CAD build for the part. Positions are in the model's coordinates, mm. A direction names the side the tool comes from. Round coordinates to 2 decimals unless told otherwise and drop trailing zeros. Loops run counter-clockwise (first coordinate to the right, second up) from the corner with the lowest first, then second, coordinate; pieces in that order, holes last. Notation, with made-up numbers: M 16,-26 L 37,-26 A19 cw 37,-20 Z; hole C 45,54 d8. An arc over 180 degrees is marked long. Put each result on its own line as item: value. Start each with the question number.
from build123d import *

# Parameters (mm, degrees)
F0_W     = 59.6908442676
F0_H     = 73.2762925327
F0_W_2   = 45.3756786883
F1_DEPTH = 38.1
F3_DEPTH = 76.2
F4_W     = 20.4342082143
F4_H     = 8.8877151668
F5_DEPTH = 76.2
F6_W     = 27.9634296894
F6_H     = 14.7078186274
F7_DEPTH = 25.4
F8_R     = 4.8926994205
F8_R_2   = 4.9486448894
F8_R_3   = 4.9129402175
F8_R_4   = 5.3604581345
F9_DEPTH = 76.2


with BuildPart() as f1:
    # F0 (on Top) → F1 (new body)
    with BuildSketch(Plane.XY):
        with Locations((-29.8454221338, -36.6381462663)):
            Rectangle(F0_W, F0_H)
        with Locations((22.6878393441, -36.6381462663)):
            Rectangle(F0_W_2, F0_H)
    extrude(amount=F1_DEPTH)

    # F2 (on Front) → F3 (cut)
    with BuildSketch(Plane.XZ):
        Polygon((-9.0658813715, 42.4513481557), (46.1928248405, 0), (48.2074655592, 0), (48.2074655592, 42.4513481557), align=None)
    extrude(amount=F3_DEPTH, mode=Mode.SUBTRACT)

    # F4 (on face) → F5 (cut)
    with BuildSketch(Plane(origin=(-59.6908442676, 0, 0), x_dir=(0, -1, 0), z_dir=(-1, 0, 0))):
        with Locations((37.7025529742, 33.6561424166)):
            Rectangle(F4_W, F4_H)
    extrude(amount=-F5_DEPTH, mode=Mode.SUBTRACT)

    # F6 (on face) → F7 (cut)
    with BuildSketch(Plane(origin=(0, 0, 0), x_dir=(1, 0, 0), z_dir=(0, 0, -1))):
        with Locations((31.3939638436, 65.922383219)):
            Rectangle(F6_W, F6_H)
    extrude(amount=-F7_DEPTH, mode=Mode.SUBTRACT)

    # F8 (on face) → F9 (cut)
    with BuildSketch(Plane(origin=(0, 0, 0), x_dir=(1, 0, 0), z_dir=(0, 0, -1))):
        with Locations((12.5195495784, 40.1489026845)):
            Circle(F8_R)
        with Locations((12.4636041095, 14.2439040613)):
            Circle(F8_R_2)
        with Locations((32.2204525995, 40.1489026845)):
            Circle(F8_R_3)
        with Locations((32.3233206043, 13.9583635985)):
            Circle(F8_R_4)
    extrude(amount=-F9_DEPTH, mode=Mode.SUBTRACT)


solid = f1.part
(1) Cut at C-C on z = 3.5. List the corners of the cut face in (x, y), and give its area (3 significant figures).
(2) Cut at B-B on y = -54. List the corners of the cut face in (x, z), and give its area (3 significant figures).
(3) Tool access for faces 4 (the flat face through (-8, -36, 0)), 5 (the flat face through (-26, -27.485, 34)), 6 (the flat face through (28, -58.568, 8)): list every direction of +Z, -Z, +X, -X, +Y, -Y with a clear straight run to the whole face (end or side of a thin tool).
(4) Cut at A-A on x = 30. List the corners of the cut face in (y, z).
(5) Cut at D-D on x = -35. List the corners of the cut face in (y, z).
(6) Mould opens along X. For faces 1 (the flat face through (-22, -73.276, 19)), 2 (the flat face through (17.412, -66, 11)), 3 (the cylindrical face through (7.52, -14.46, 11.41)) say: +X half, -X half, draft (parallel to the pull), parting line (faces both ways), or undercut.
(7) Drill centre lines: line 1 along Y through (x, z) = (-52, 35); line 2 along X through (y, z) = (-10, 4.5); line 3 along Y through (x, z) = (24, 7). Where is each one in solid material? Low to high.
(8) Flat gauge pins, fed straight in: pin 1 Ø15.5 at (x, y) = (32.22, -40.15) entering from -Z; pin 2 Ø4 at (x, y) = (30, -32) entering from +Z; pin 3 Ø17.5 at (x, z) = (31.5, 5.5) entering from -Y; pin 4 Ø4 at (x, y) = (-18, -42) entering from +Z. Where does each tip first touch, or does it go through?
Taken from the geometry:
1. outline: M -59.69,-73.28 L 17.41,-73.28 L 17.41,-58.57 L 41.64,-58.57 L 41.64,0 L -59.69,0 Z; hole C 12.46,-14.24 d9.9; hole C 12.52,-40.15 d9.79; hole C 32.32,-13.96 d10.72; hole C 32.22,-40.15 d9.83
1. area: 6,750 mm2
2. outline: M -59.69,0 L 45.38,0 L 45.38,0.63 L -3.4,38.1 L -59.69,38.1 Z
2. area: 3,090 mm2
3. face 4: -Z, +X, -X, +Y, -Y
3. face 5: +Z, +X, -X
3. face 6: +Z, -Z, +X, -Y
4. outline: M -58.57,0 L -44.53,0 L -44.53,12.44 L -58.57,12.44 Z; M -35.77,0 L -18.79,0 L -18.79,12.44 L -35.77,12.44 Z; M -9.13,0 L 0,0 L 0,12.44 L -9.13,12.44 Z
5. outline: M -73.28,0 L 0,0 L 0,38.1 L -27.49,38.1 L -27.49,29.21 L -47.92,29.21 L -47.92,38.1 L -73.28,38.1 Z
6. face 1: draft
6. face 2: +X half
6. face 3: undercut
7. line 1: -73.28 to -47.92, -27.49 to 0
7. line 2: -59.69 to 9.92, 15.01 to 28.71, 35.94 to 40.34
7. line 3: -58.57 to 0
8. pin 1: z = 0
8. pin 2: z = 13.98
8. pin 3: y = -58.57
8. pin 4: z = 29.21
